Design review of the part shown in the three views and the two pictorial views. Dimensions are in mm from the part's minimum x, y and z. Coordinates: 2 decimals unless noted, no trailing zeros. Write each loop counter-clockwise with the first axis right and the second up, starting at its lowest first coordinate (ties: lowest second). Pieces come first, ordered by that corner, then holes.
Q1. Take a section at A-A, the plane y = 168.5. Write out the cut boundary in (x, z).
Q2. Take a section at B-B, the plane z = 126. Write out the cut boundary in (x, y), plus the area to 3 significant figures.
Q3. Take a section at C-C, the plane x = 1.15. State how many separate pieces and enclosed holes the cut face has, plus the area to 3 significant figures.
Q4. For pin 1 Ø3 at (x, z) = (4, 77) entering from +Y; pin 2 Ø3 at (y, z) = (5, 94.5) entering from +X; pin 3 Ø1 at (x, z) = (3.5, 43.5) entering from +Y (3 decimals), all flat-tipped, find the tip position at first contact; note any pin that passes through.
Q5. For L1, parallel to Y at x = 1.5, z = 94.5; L2, parallel to Y at x = 0.3, z = 75.5; L3, parallel to Y at x = 1.3, z = 22.5, list the stretches that pass through material, from the lowest coordinate up.
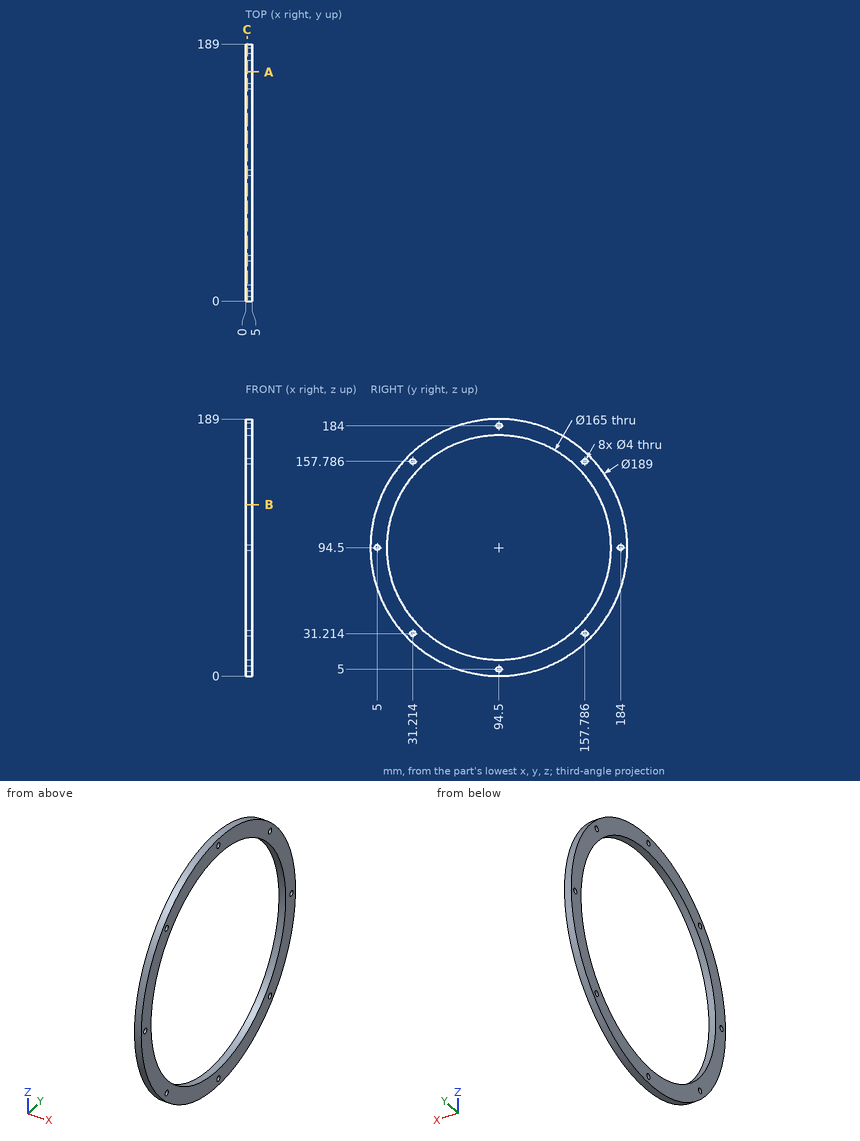
Responses:
1. outline: (0, 35.73) - (5, 35.73) - (5, 58.03) - (0, 58.03) - close; (0, 130.97) - (5, 130.97) - (5, 153.27) - (0, 153.27) - close
2. outline: (0, 5.4) - (5, 5.4) - (5, 18.25) - (0, 18.25) - close; (0, 170.75) - (5, 170.75) - (5, 183.6) - (0, 183.6) - close
2. area: 128 mm2
3. separate pieces: 1
3. enclosed holes: 9
3. area: 6,570 mm2
4. pin 1: stops at y = 187.64
4. pin 2: passes through
4. pin 3: stops at y = 174.375
5. L1: y = 0 to 3, 7 to 12, 177 to 182, 186 to 189
5. L2: y = 1.93 to 14.22, 174.78 to 187.07
5. L3: y = 33.29 to 54.22, 134.78 to 155.71
